Autodesk Fusion 360 part; units mm, degrees
sketch "Sketch1" plane through (0, 0, 0) normal (0, 0, 1) x (1, 0, 0)
  line L0 (-45, 60) -> (45, 60)
  line L1 (45, 60) -> (45, -60)
  line L2 (45, -60) -> (-45, -60)
  line L3 (-45, -60) -> (-45, 60)
  line L4 (-45, 60) -> (45, -60) construction
  line L5 (45, 60) -> (-45, -60) construction
  dimension "d1" = 90
  dimension "d2" = 120
sketch "Sketch3" plane through (0, 0, 0) normal (0, 0, 1) x (1, 0, 0)
  line L0 (-47.5, 65) -> (47.5, 65)
  line L1 (47.5, 65) -> (47.5, -65)
  line L2 (47.5, -65) -> (-47.5, -65)
  line L3 (-47.5, -65) -> (-47.5, 65)
  line L4 (-47.5, 65) -> (47.5, -65) construction
  line L5 (47.5, 65) -> (-47.5, -65) construction
  dimension "d8" = 95
  dimension "d9" = 130
extrude "Extrude3" add sketch "Sketch3" along normal blind 5
sketch "Sketch4" plane through (0, 0, 5) normal (0, 0, 1) x (-1, 0, 0)
  line L0 (47.5, 65) -> (-47.5, 65)
  line L1 (-47.5, 65) -> (-47.5, -65)
  line L2 (-47.5, -65) -> (47.5, -65)
  line L3 (47.5, -65) -> (47.5, 65)
  circle A0 centre (0, 36.6491) radius 20
  dimension "d12" = 40
extrude "Extrude4" cut sketch "Sketch4" against normal blind 10 contours A0
sketch "Sketch5" plane through (0, 0, 5) normal (0, 0, 1) x (-1, 0, 0)
  circle A0 centre (0, 36.6491) radius 20
  line L0 (47.5, 65) -> (-47.5, 65)
  line L1 (-47.5, 65) -> (-47.5, -65)
  line L2 (-47.5, -65) -> (47.5, -65)
  line L3 (47.5, -65) -> (47.5, 65)
  line L4 (47.5, -65) -> (42.5, -65)
  line L5 (42.5, -65) -> (42.5, 65)
  line L6 (42.5, 65) -> (47.5, 65)
  line L7 (47.5, 65) -> (47.5, -65)
  dimension "d15" = 5
extrude "Extrude5" add sketch "Sketch5" along normal blind 60 contours L0 L2 L3 L4 L5 L6 L7
fillet "Fillet1" radius 2 1 edges at (-42.5, 0, 5)
sketch "Sketch6" plane through (-42.5, 0, 0) normal (1, 0, 0) x (0, 1, 0)
  line L0 (-65, 7) -> (65, 7)
  line L1 (65, 7) -> (65, 65)
  line L2 (65, 65) -> (-65, 65)
  line L3 (-65, 65) -> (-65, 7)
  circle A0 centre (-50, 50) radius 5
  circle A1 centre (50, 50) radius 5
  dimension "d20" = 10
  dimension "d21" = 10
extrude "Extrude6" cut sketch "Sketch6" against normal blind 10 contours A0
sketch "Sketch7" plane through (-42.5, 0, 0) normal (1, 0, 0) x (0, 1, 0)
  circle A0 centre (-50, 50) radius 5
  line L0 (-65, 7) -> (65, 7)
  line L1 (65, 7) -> (65, 65)
  line L2 (65, 65) -> (-65, 65)
  line L3 (-65, 65) -> (-65, 7)
  circle A1 centre (50, 50) radius 5
  dimension "d24" = 10
extrude "Extrude7" cut sketch "Sketch7" against normal blind 20 contours A1
sketch "Sketch8" plane through (0, 0, 5) normal (0, 0, 1) x (-1, 0, 0)
  line L0 (40.5, -65) -> (40.5, 65)
  line L1 (40.5, 65) -> (-47.5, 65)
  line L2 (-47.5, 65) -> (-47.5, -65)
  line L3 (-47.5, -65) -> (40.5, -65)
  circle A0 centre (0, 36.6491) radius 20
  line L4 (-47.5, -10.1158) -> (-42.5, -10.1158)
  line L5 (-42.5, -10.1158) -> (-42.5, -65)
  line L6 (-42.5, -65) -> (-47.5, -65)
  line L7 (-47.5, -65) -> (-47.5, -10.1158)
  dimension "d27" = 5
extrude "Extrude8" add sketch "Sketch8" along normal blind 20 contours L2 L3 L4 L5 L6 L7
fillet "Fillet2" radius 1 1 edges at (42.5, 37.5579, 5)
extrude "Extrude1" [suppressed]
sketch "Sketch2" plane through (0, 0, 5) normal (0, 0, 1) x (-1, 0, 0)
  line L0 (45, 60) -> (-45, 60)
  line L1 (-45, 60) -> (-45, -60)
  line L2 (-45, -60) -> (45, -60)
  line L3 (45, -60) -> (45, 60)
  circle A0 centre (0, 0) radius 20
  dimension "d5" = 40
extrude "Extrude2" [suppressed]
Build history of the part. All positions in model axes, mm. A direction names the side the tool comes from. Give positions to 0.01 mm unless a question says otherwise; leave off trailing zeros. Order: outer loops, then holes, each group sorted by start corner. A loop starts at its lowest first (then second) coordinate and runs counter-clockwise, first axis right, second up. Notation, with made-up numbers: M -20.75,43 L 6.25,43 A22 cw 6.25,80 Z; hole C -10,-15.75 d11. An arc over 180 degrees is marked long. Write item = value, one per line. Start each with the question number.
(1) Slice it at D-D on y = -6. Write the cut outline in (x, z), plus the area to 3 significant figures.
(2) Probe L1, parallel to Y at x = 0, z = 2.2; L2, parallel to X at y = 26.5, z = 24; L3, parallel to Z at x = 11, y = 56. List the from-to ranges inside material, lowest first. Write a range as [from, to].
(3) Slice it at C-C on z = 50. Write the cut outline in (x, y).
(4) Which spindle directions (+Z, -Z, +X, -X, +Y, -Y) get a long thin tool onto all of the face, cutting with end or side? Do faces 1 (the flat face through (-10, 65, 3)), 2 (the flat face through (45, 10.116, 15)), 3 (the flat face through (45, 37, 25)), 4 (the flat face through (-47.5, 1, 32)), 5 (the flat face through (42.5, 37, 15)). Say none if no direction does.
(5) Slice it at B-B on y = 50. Write the cut outline in (x, z).
(6) Pin check, flat tips, straight feed: pin 1 Ø3 at (x, z) = (43.5, 11) entering from -Y; pin 2 Ø3 at (x, y) = (17, 43.5) entering from +Z; pin 3 Ø5.5 at (x, y) = (45, 51) entering from +Z; pin 4 Ø12 at (x, y) = (-36.5, 2) entering from -Z. Stop position of each tip, or through.
(7) Slice it at A-A on x = 0. Write the cut outline in (y, z), plus the area to 3 significant figures.
(8) Two-plate mould, pull along Z, no slides. Class faces 6 (the cylindrical face through (-44.965, -50.651, 54.957)), 7 (the flat face through (-1, 1, 0)), 8 (the cylindrical face through (-19.076, -42.657, 2.535)): released by +Z, released by -Z, zero draft, split by the parting line, or undercut.
Responses:
q1.outline = M -47.5,0 L 47.5,0 L 47.5,5 L -40.5,5 A2 cw -42.5,7 L -42.5,65 L -47.5,65 Z
q1.area = 776 mm2
q2.L1 = [-65, -56.65], [-16.65, 65]
q2.L2 = [-47.5, -42.5], [42.5, 47.5]
q2.L3 = [0, 5]
q3.outline = M -47.5,-65 L -42.5,-65 L -42.5,-55 L -47.5,-55 Z; M -47.5,-45 L -42.5,-45 L -42.5,45 L -47.5,45 Z; M -47.5,55 L -42.5,55 L -42.5,65 L -47.5,65 Z
q4.face_1 = +Z, -Z, +X, -X, +Y
q4.face_2 = +Z, +X, -Y
q4.face_3 = +Z, +X, +Y, -Y
q4.face_4 = +Z, -Z, -X, +Y, -Y
q4.face_5 = +Z, +Y, -Y
q5.outline = M -47.5,0 L 47.5,0 L 47.5,25 L 42.5,25 L 42.5,6 A1 cw 41.5,5 L -40.5,5 A2 cw -42.5,7 L -42.5,45 L -47.5,45 Z; M -47.5,55 L -42.5,55 L -42.5,65 L -47.5,65 Z
q6.pin_1 = 10.12
q6.pin_2 = 5
q6.pin_3 = 25
q6.pin_4 = 0
q7.outline = M -65,0 L -56.65,0 L -56.65,5 L -65,5 Z; M -16.65,0 L 65,0 L 65,5 L -16.65,5 Z
q7.area = 450 mm2
q8.face_6 = undercut
q8.face_7 = released by -Z
q8.face_8 = zero draft
